Geometry: final body of the model. Coordinates: model frame, mm. A direction names the side the tool comes from. Coordinates: 2 decimals unless noted, no trailing zeros. Write each loop counter-clockwise with the first axis right and the second up, starting at its lowest first coordinate (ties: lowest second). Pieces come first, ordered by that corner, then holes. Notation, with made-up numbers: (-22, 46.5) -> (28, 46.5) arc R17 ccw to (28, 75.5) -> close; hole circle Ø4 at (-6, -26.5). An arc over 180 degrees is marked (long way). One line per item, written item: value.
```python
from build123d import *

# Parameters (mm, degrees)
SKETCH1_W               = 91
SKETCH1_H               = 50
BOSS_EXTRUDE1_DEPTH     = 12
SKETCH2_W               = 18
SKETCH2_H               = 50
BOSS_EXTRUDE2_DEPTH     = 28
SKETCH4_W               = 50
SKETCH4_H               = 12
BOSS_EXTRUDE3_DEPTH     = 49.5
SKETCH5_W               = 50
SKETCH5_H               = 12
BOSS_EXTRUDE4_DEPTH     = 49.5
CUT_EXTRUDE1_DEPTH      = 29
CUT_EXTRUDE1_DEPTH_BACK = 13
CUT_EXTRUDE2_DEPTH      = 29
CUT_EXTRUDE2_DEPTH_BACK = 13
SKETCH9_W               = 18
SKETCH9_H               = 50
BOSS_EXTRUDE5_DEPTH     = 58
SKETCH10_R              = 8
CUT_EXTRUDE3_DEPTH      = 50.5
CUT_EXTRUDE3_DEPTH_BACK = 141.5
SKETCH12_R              = 5.769053465
SKETCH12_R_2            = 7.5
CUT_EXTRUDE4_DEPTH      = 59
CUT_EXTRUDE4_DEPTH_BACK = 41
SKETCH15_W              = 55
SKETCH15_H              = 8
BOSS_EXTRUDE6_DEPTH     = 28


with BuildPart() as part:
    # Sketch1 → Boss-Extrude1 (new body)
    with BuildSketch(Plane(origin=(0, 0, 0), x_dir=(1, 0, 0), z_dir=(0, 1, 0))):
        Rectangle(SKETCH1_W, SKETCH1_H)
    extrude(amount=-BOSS_EXTRUDE1_DEPTH)

    # Sketch2 → Boss-Extrude2 (add)
    with BuildSketch(Plane.XZ.offset(12)):
        with Locations((-36.5, 0)):
            Rectangle(SKETCH2_W, SKETCH2_H)
        with Locations((36.5, 0)):
            Rectangle(SKETCH2_W, SKETCH2_H)
    extrude(amount=BOSS_EXTRUDE2_DEPTH)

    # Sketch4 → Boss-Extrude3 (add)
    with BuildSketch(Plane(origin=(45.5, 0, 0), x_dir=(0, 0, -1), z_dir=(1, 0, 0))):
        with Locations((0, -34)):
            Rectangle(SKETCH4_W, SKETCH4_H)
    extrude(amount=BOSS_EXTRUDE3_DEPTH)

    # Sketch5 → Boss-Extrude4 (add)
    with BuildSketch(Plane.ZY.offset(45.5)):
        with Locations((0, -34)):
            Rectangle(SKETCH5_W, SKETCH5_H)
    extrude(amount=BOSS_EXTRUDE4_DEPTH)

    # Sketch7 → Cut-Extrude1 (cut, two sides)
    with BuildSketch(Plane(origin=(0, -28, 0), x_dir=(1, 0, 0), z_dir=(0, 1, 0))) as cut_extrude1_sk:
        Polygon((95, -25), (95, -5), (70, -25), align=None)
    extrude(amount=CUT_EXTRUDE1_DEPTH, mode=Mode.SUBTRACT)
    extrude(cut_extrude1_sk.sketch, amount=-CUT_EXTRUDE1_DEPTH_BACK, mode=Mode.SUBTRACT)

    # Sketch8 → Cut-Extrude2 (cut, two sides)
    with BuildSketch(Plane(origin=(0, -28, 0), x_dir=(1, 0, 0), z_dir=(0, 1, 0))) as cut_extrude2_sk:
        Polygon((-95, -25), (-95, -5), (-70, -25), align=None)
    extrude(amount=CUT_EXTRUDE2_DEPTH, mode=Mode.SUBTRACT)
    extrude(cut_extrude2_sk.sketch, amount=-CUT_EXTRUDE2_DEPTH_BACK, mode=Mode.SUBTRACT)

    # Sketch9 → Boss-Extrude5 (add)
    with BuildSketch(Plane(origin=(0, 0, 0), x_dir=(1, 0, 0), z_dir=(0, 1, 0))):
        with Locations((-36.5, 0)):
            Rectangle(SKETCH9_W, SKETCH9_H)
        with Locations((36.5, 0)):
            Rectangle(SKETCH9_W, SKETCH9_H)
    extrude(amount=BOSS_EXTRUDE5_DEPTH)

    # Sketch10 → Cut-Extrude3 (cut, two sides)
    with BuildSketch(Plane(origin=(45.5, 0, 0), x_dir=(0, 0, -1), z_dir=(1, 0, 0))) as cut_extrude3_sk:
        with BuildLine():
            Line((25, 58), (0, 58))
            ThreePointArc((0, 58), (13.247648854, 55.742546282), (25, 49.224989992))
            Line((25, 49.224989992), (25, 58))
        make_face()
        with BuildLine():
            Line((-25, 58), (-25, 49.224989992))
            ThreePointArc((-25, 49.224989992), (-13.247648854, 55.742546282), (0, 58))
            Line((0, 58), (-25, 58))
        make_face()
        with Locations((0, 18)):
            Circle(SKETCH10_R)
    extrude(amount=CUT_EXTRUDE3_DEPTH, mode=Mode.SUBTRACT)
    extrude(cut_extrude3_sk.sketch, amount=-CUT_EXTRUDE3_DEPTH_BACK, mode=Mode.SUBTRACT)

    # Sketch12 → Cut-Extrude4 (cut, two sides)
    with BuildSketch(Plane(origin=(0, 0, 0), x_dir=(1, 0, 0), z_dir=(0, 1, 0))) as cut_extrude4_sk:
        with Locations((77.5, 7)):
            Circle(SKETCH12_R)
        with Locations((-77.5, 7)):
            Circle(SKETCH12_R_2)
    extrude(amount=CUT_EXTRUDE4_DEPTH, mode=Mode.SUBTRACT)
    extrude(cut_extrude4_sk.sketch, amount=-CUT_EXTRUDE4_DEPTH_BACK, mode=Mode.SUBTRACT)

    # Sketch15 → Boss-Extrude6 (add)
    with BuildSketch(Plane.XZ.offset(12)):
        with Locations((0, -7)):
            Rectangle(SKETCH15_W, SKETCH15_H)
    extrude(amount=BOSS_EXTRUDE6_DEPTH)


solid = part.part
```
(1) Line query: line 1 (X direction, y = -30, z = -7); line 2 (X direction, y = -26, z = 17.5); line 3 (Y direction, x = 20.5, z = 6.5). Output: solid intervals per line, ascending. Write a range as [from, to].
Responses:
line 1: x = [-95, -85], [-70, 71.73], [83.27, 95]
line 2: x = [-45.5, -27.5], [27.5, 45.5]
line 3: y = [-12, 0]
(2) Reachability of faces 5 (the flat face through (45.5, 6, 0)), 6 (the flat face through (0, -26, -3)), 7 (the flat face through (27.5, 29, 0)) from +Z, -Z, +X, -X, +Y, -Y: full face, straight path, thin tool, end or side. Return the list, or none.
Responses:
face 5: +Z, -Z, +X, +Y
face 6: +Z, -Y
face 7: +Z, -Z, +Y
(3) Section C-C (y = 18). Return the cut outline in (x, z), then the cut area to 3 significant figures.
Responses:
outline: (-45.5, -25) -> (-27.5, -25) -> (-27.5, -8) -> (-45.5, -8) -> close; (-45.5, 8) -> (-27.5, 8) -> (-27.5, 25) -> (-45.5, 25) -> close; (27.5, -25) -> (45.5, -25) -> (45.5, -8) -> (27.5, -8) -> close; (27.5, 8) -> (45.5, 8) -> (45.5, 25) -> (27.5, 25) -> close
area: 1,220 mm2
(4) Section B-B (y = 39.5). Return the cut outline in (x, z).
Responses:
outline: (-45.5, -25) -> (-27.5, -25) -> (-27.5, 25) -> (-45.5, 25) -> close; (27.5, -25) -> (45.5, -25) -> (45.5, 25) -> (27.5, 25) -> close
(5) Section D-D (x = -4). Return the cut outline in (y, z), then the cut area to 3 significant figures.
Responses:
outline: (-40, -11) -> (-12, -11) -> (-12, -25) -> (0, -25) -> (0, 25) -> (-12, 25) -> (-12, -3) -> (-40, -3) -> close
area: 824 mm2
(6) Pull-direction query (Z, two-part tool) for faces 1 (the flat face through (0, -26, -11)), 2 (the cylindrical face through (83.003, -33.916, -8.733)), 3 (the flat face through (70, -28, 0)), 4 (the flat face through (-6, -2, 25)); classes: released by +Z, released by -Z, zero draft, split by the parting line, or undercut.
Responses:
face 1: released by -Z
face 2: undercut
face 3: zero draft
face 4: released by +Z
(7) First-contact query: pin 1 (15 mm diameter, centred on y = 0.5, z = 1.5, fed in from +X); pin 2 (8.5 mm diameter, centred on y = -29.5, z = 15, fed in from -X); pin 3 (8.5 mm diameter, centred on x = 10, y = -24.5, fed in from -Z). Flat tips, straight axial feed; report the tip coordinate or a pass-through.
Responses:
pin 1: stops at x = 45.5
pin 2: stops at x = -87.81
pin 3: stops at z = -11
(8) Section A-A (x = -77.5). Return the cut outline in (y, z), then the cut area to 3 significant figures.
Responses:
outline: (-40, -25) -> (-28, -25) -> (-28, -14.5) -> (-40, -14.5) -> close; (-40, 0.5) -> (-28, 0.5) -> (-28, 19) -> (-40, 19) -> close
area: 348 mm2
